Check sheet for the modelled part. Datum: model origin and axes. Units: mm. Face numbers are marked on the shaded views. A direction names the side the tool comes from. Give positions to 0.01 mm unless a question says otherwise; leave off trailing zeros. Order: outer loops, then holes, each group sorted by start corner. A loop starts at its lowest first (then second) coordinate and runs counter-clockwise, first axis right, second up. Notation, with made-up numbers: (46.5, -9) - (61.5, -9) arc R24 cw to (61.5, 25) - close; hole circle Ø7 at (9.25, -17.5). An arc over 180 degrees is marked (long way). Answer in a Markdown table with one row per item.
from build123d import *

# Parameters (mm, degrees)
SKETCH1_R           = 13
SKETCH1_R_2         = 8
BOSS_EXTRUDE2_DEPTH = 10
CUT_EXTRUDE1_START  = -1.5
CUT_EXTRUDE1_DEPTH  = 1.5
CUT_EXTRUDE2_DEPTH  = 1.5


with BuildPart() as part:
    # Sketch1 → Boss-Extrude2 (new body)
    with BuildSketch(Plane(origin=(0, 0, 0), x_dir=(1, 0, 0), z_dir=(0, 1, 0))):
        with BuildLine():
            ThreePointArc((1.730769231, 22.433333187), (-22.5, 0), (1.730769231, -22.433333187))
            Line((1.730769231, -22.433333187), (130.961538462, -12.462962882))
            ThreePointArc((130.961538462, -12.462962882), (142.5, 0), (130.961538462, 12.462962882))
            Line((130.961538462, 12.462962882), (1.730769231, 22.433333187))
        make_face()
        with Locations(Location((0, 0, 0), (0, 0, 270))):
            Circle(SKETCH1_R, mode=Mode.SUBTRACT)
        with Locations(Location((130, 0, 0), (0, 0, 270))):
            Circle(SKETCH1_R_2, mode=Mode.SUBTRACT)
    extrude(amount=BOSS_EXTRUDE2_DEPTH)

    # Sketch3 → Cut-Extrude1 (cut)
    with BuildSketch(Plane(origin=(0, 10, 0), x_dir=(1, 0, 0), z_dir=(0, 1, 0)).offset(CUT_EXTRUDE1_START)):
        with BuildLine():
            Line((15.446386754, 16.360291448), (120.606552772, 8.247008498))
            ThreePointArc((120.606552772, 8.247008498), (117.5, 0), (120.606552772, -8.247008498))
            Line((120.606552772, -8.247008498), (15.446386754, -16.360291448))
            ThreePointArc((15.446386754, -16.360291448), (22.5, 0), (15.446386754, 16.360291448))
        make_face()
    extrude(amount=CUT_EXTRUDE1_DEPTH, mode=Mode.SUBTRACT)

    # Sketch5 → Cut-Extrude2 (cut)
    with BuildSketch(Plane.XZ):
        with BuildLine():
            Line((15.446386754, 16.360291448), (120.606552772, 8.247008498))
            ThreePointArc((120.606552772, 8.247008498), (117.5, 0), (120.606552772, -8.247008498))
            Line((120.606552772, -8.247008498), (15.446386754, -16.360291448))
            ThreePointArc((15.446386754, -16.360291448), (22.5, 0), (15.446386754, 16.360291448))
        make_face()
    extrude(amount=-CUT_EXTRUDE2_DEPTH, mode=Mode.SUBTRACT)


solid = part.part
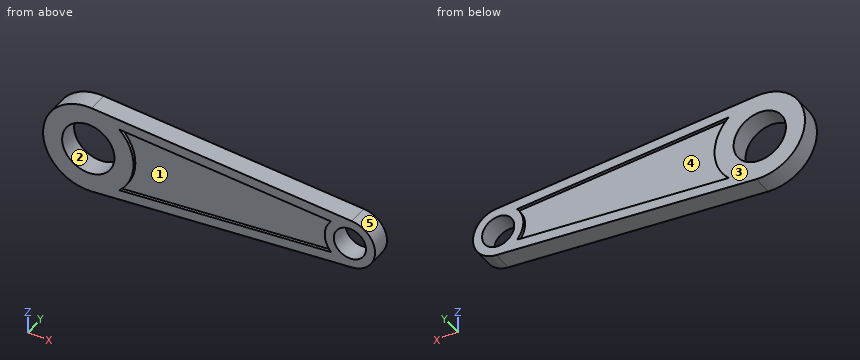
(1) Cross-section at C-C, the plane y = 6. Record the cut outline in (x, z).
Geometry says:
| item | result |
|---|---|
| outline | (1.73, -22.43) - (130.96, -12.46) arc R12.5 ccw to (130.96, 12.46) - (1.73, 22.43) arc R22.5 ccw (long way) to start; hole circle Ø26 at (0, 0); hole circle Ø16 at (130, 0) |
(2) Cross-section at D-D, the plane z = -11. Record the cut outline in (x, y).
Geometry says:
| item | result |
|---|---|
| outline | (-19.63, 0) - (-6.93, 0) - (-6.93, 10) - (-19.63, 10) - close; (6.93, 0) - (19.63, 0) - (19.63, 1.5) - (84.92, 1.5) - (84.92, 0) - (135.94, 0) - (135.94, 10) - (84.92, 10) - (84.92, 8.5) - (19.63, 8.5) - (19.63, 10) - (6.93, 10) - close |
(3) Gauge pin test, flat ends, axial feed: P1, Ø3, axis at y = 4.5, z = 13.5, coming from the -X side; P2, Ø6, axis at y = 6.5, z = -14.5, coming from the +X side; P3, Ø9.5, axis at x = 130, z = 0, coming from the -Y side; P4, Ø1.5, axis at x = 56, z = -2.5, coming from the +Y side. Record the tip position at first contact, or that the pin passes through.
Geometry says:
| item | result |
|---|---|
| P1 | x = -19.03 |
| P2 | x = 134.9 |
| P3 | through |
| P4 | y = 8.5 |
(4) Access from +Z, -Z, +X, -X, +Y, -Y to the whole of each face (thin tool, end or side, straight path). Record for the marked faces 1 and 2.
Geometry says:
| item | result |
|---|---|
| face 1 | -Y |
| face 2 | +Y, -Y |
(5) Cross-section at A-A, the plane x = 0. Record the cut outline in (y, z), then the cut area to 3 significant figures.
Geometry says:
| item | result |
|---|---|
| outline | (0, -22.5) - (10, -22.5) - (10, -13) - (0, -13) - close; (0, 13) - (10, 13) - (10, 22.5) - (0, 22.5) - close |
| area | 190 mm² |
(6) Cross-section at B-B, the plane z = 0. Record the cut outline in (x, y).
Geometry says:
| item | result |
|---|---|
| outline | (-22.5, 0) - (-13, 0) - (-13, 10) - (-22.5, 10) - close; (13, 0) - (22.5, 0) - (22.5, 1.5) - (117.5, 1.5) - (117.5, 0) - (122, 0) - (122, 10) - (117.5, 10) - (117.5, 8.5) - (22.5, 8.5) - (22.5, 10) - (13, 10) - close; (138, 0) - (142.5, 0) - (142.5, 10) - (138, 10) - close |
(7) Mould release check, pull along X, two halves, no side actions. Record for the marked faces 3, 4 and 5: pulls with the +X half, pulls with the -X half, needs draft (parallel to the pull), parting line crosses it, or undercut.
Geometry says:
| item | result |
|---|---|
| face 3 | needs draft |
| face 4 | undercut |
| face 5 | pulls with the +X half |
(8) Thickness scan on L1, parallel to X at y = 4, z = 0; L2, parallel to Y at x = 77, z = 8.5; L3, parallel to X at y = 4.5, z = -5.5. Record the ranges inside material, lowest first.
Geometry says:
| item | result |
|---|---|
| L1 | -22.5 to -13, 13 to 122, 138 to 142.5 |
| L2 | 1.5 to 8.5 |
| L3 | -21.82 to -11.78, 11.78 to 124.19, 135.81 to 141.22 |
